```python
from build123d import *

# Parameters (mm, degrees)
SKETCH1_W           = 314.4612
SKETCH1_H           = 3.175
BOSS_EXTRUDE1_DEPTH = 200.66180012
CUT_EXTRUDE2_START  = -3.175
SKETCH5_W           = 3.175
SKETCH5_H           = 86.36
CUT_EXTRUDE2_DEPTH  = 259.119504214
SKETCH3_W           = 80
SKETCH3_H           = 3.175
BOSS_EXTRUDE2_DEPTH = 3.175
LPATTERN2_COUNT     = 2
LPATTERN2_PITCH     = 154.43
BOSS_EXTRUDE3_DEPTH = 3.175


with BuildPart() as part:
    # Sketch1 → Boss-Extrude1 (new body)
    with BuildSketch(Plane.XY):
        Rectangle(SKETCH1_W, SKETCH1_H)
    extrude(amount=BOSS_EXTRUDE1_DEPTH)

    # Sketch5 → Cut-Extrude2 (cut)
    with BuildSketch(Plane(origin=(0, 1.5875, 0), x_dir=(1, 0, 0), z_dir=(0, 1, 0)).offset(CUT_EXTRUDE2_START)):
        with Locations((-155.6431, -157.48180012)):
            Rectangle(SKETCH5_W, SKETCH5_H)
    cut_extrude2 = extrude(amount=CUT_EXTRUDE2_DEPTH, mode=Mode.SUBTRACT)

    # Mirror1: Cut-Extrude2 across plane
    add(cut_extrude2.mirror(Plane(origin=(0, 0, 0), x_dir=(0, 0, 1), z_dir=(1, 0, 0))), mode=Mode.SUBTRACT)

    # Sketch3 → Boss-Extrude2 (add)
    with BuildSketch(Plane(origin=(0, 0, 0), x_dir=(-1, 0, 0), z_dir=(0, 0, -1))):
        with Locations((-77.2306, 0)):
            Rectangle(SKETCH3_W, SKETCH3_H)
    boss_extrude2 = extrude(amount=BOSS_EXTRUDE2_DEPTH)

    # LPattern2: Boss-Extrude2 ×2
    with Locations(*[(-i * LPATTERN2_PITCH, 0, 0) for i in range(1, LPATTERN2_COUNT)]):
        add(boss_extrude2)

    # Sketch10 → Boss-Extrude3 (add)
    with BuildSketch(Plane.XZ.offset(1.5875)):
        Polygon((201.66536, 0), (201.66536, 3.175), (160.4056, 50.8), (157.2306, 50.8), (157.2306, 0), align=None)
    extrude(amount=-BOSS_EXTRUDE3_DEPTH)


solid = part.part
```
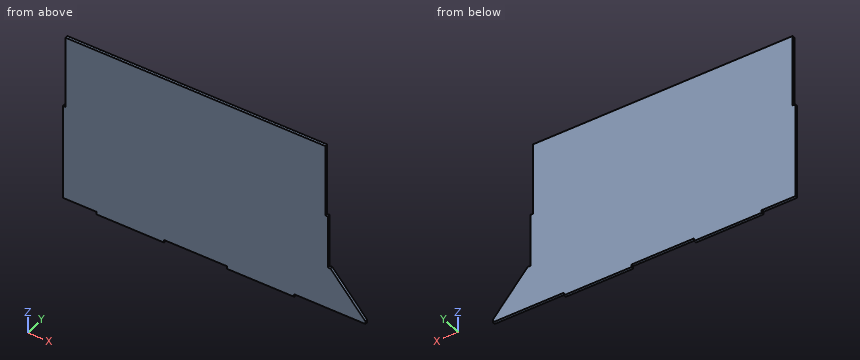
Can you work these out from the model? Positions are in its coordinate system, mm. Round coordinates to 2 decimals unless told otherwise and drop trailing zeros. Loops run counter-clockwise (first coordinate to the right, second up) from the corner with the lowest first, then second, coordinate; pieces in that order, holes last. Notation, with made-up numbers: M 4,74 L 56,74 A24 ccw 56,101 Z; hole C 12,38 d10. An arc over 180 degrees is marked long. Answer in a Markdown table with one row per item.
1. I'm going to push flat-ended pins straight in: pin 1 Ø1.5 at (y, z) = (1, 25.5) entering from +X; pin 2 Ø1 at (x, y) = (-1.5, -0.5) entering from -Z; pin 3 Ø1 at (y, z) = (0.5, 156.5) entering from -X. Where does each tip first touch, or does it pass through?
Established:
| item | result |
|---|---|
| pin 1 | x = 182.97 |
| pin 2 | z = 0 |
| pin 3 | x = -154.06 |
2. If we section it at C-C, the plane z = 56.5: Please give me the cut outline in (x, y).
Established:
| item | result |
|---|---|
| outline | M -157.23,-1.59 L 157.23,-1.59 L 157.23,1.59 L -157.23,1.59 Z |
3. If we section it at B-B, the plane x = 148: Please give me the cut outline in (y, z).
Established:
| item | result |
|---|---|
| outline | M -1.59,0 L 1.59,0 L 1.59,200.66 L -1.59,200.66 Z |
4. If we section it at A-A, the plane y = 0.2: Please give me the cut outline in (x, z) (3 decimals).
Established:
| item | result |
|---|---|
| outline | M -157.231,0 L -117.199,0 L -117.199,-3.175 L -37.199,-3.175 L -37.199,0 L 37.231,0 L 37.231,-3.175 L 117.231,-3.175 L 117.231,0 L 201.665,0 L 201.665,3.175 L 160.406,50.8 L 157.231,50.8 L 157.231,114.302 L 154.056,114.302 L 154.056,200.662 L -154.056,200.662 L -154.056,114.302 L -157.231,114.302 Z |
5. Please list where these lines run through material, in increasing order: line 1 (Z direction, x = 141.5, y = 0.2); line 2 (X direction, y = -1.5, z = 61); line 3 (X direction, y = 0.75, z = 166.5). Write a range as from..to.
Established:
| item | result |
|---|---|
| line 1 | 0..200.66 |
| line 2 | -157.23..157.23 |
| line 3 | -154.06..154.06 |
